Geometry check sheet. Reference: the model listing, model coordinates, mm. A direction names the side the tool comes from. Round coordinates to 2 decimals unless told otherwise and drop trailing zeros. Order: outer loops, then holes, each group sorted by start corner. A loop starts at its lowest first (then second) coordinate and runs counter-clockwise, first axis right, second up. Notation, with made-up numbers: (61, 88) - (108, 88) arc R10 cw to (108, 93) - close; hole circle Ø6 at (25.5, 6). An arc over 180 degrees is marked (long way). Answer as CSV lines item,"result". Start each with the question number.
```python
from build123d import *

# Parameters (mm, degrees)
F0_R     = 3.175
F1_DEPTH = 3.175
F2_R     = 1.5875
F3_DEPTH = 31.75
F4_R     = 3.175
F4_R_2   = 1.5875
F5_DEPTH = 3.175


with BuildPart() as f1:
    # F0 (on Front) → F1 (new body)
    with BuildSketch(Plane.XZ):
        Circle(F0_R)
    extrude(amount=F1_DEPTH)

    # F2 (on face) → F3 (join)
    with BuildSketch(Plane.XZ.offset(3.175)):
        Circle(F2_R)
    extrude(amount=F3_DEPTH)

    # F4 (on face) → F5 (join)
    with BuildSketch(Plane.XZ.offset(34.925)):
        Circle(F4_R)
        Circle(F4_R_2, mode=Mode.SUBTRACT)
        Circle(F4_R_2)
    extrude(amount=F5_DEPTH)


solid = f1.part
```
1. Thickness scan on probe 1 along Y at (x, z) = (-0.5, 1.75) (3 decimals); probe 2 along Z at (x, y) = (0, -11); probe 3 along Z at (x, y) = (1.25, -34). Record the ranges inside material, lowest first.
2. Section check A-A on x = 2.25. Record the boundary of the cut face in (y, z) (3 decimals).
3. Access from +Z, -Z, +X, -X, +Y, -Y to the whole of each face (thin tool, end or side, straight path). Record for faces 1 (the face through (-0.69, -36.49, -3.1)), 2 (the face through (1.4, -34.925, -1.4)).
4. Section check C-C on x = 0. Record the boundary of the cut face in (y, z) (1 decimal), plus the area to 3 significant figures.
5. Section check D-D on z = 0. Record the boundary of the cut face in (x, y) (1 decimal), plus the area to 3 significant figures.
6. Go/stop test with flat-tipped pins: pin 1 Ø3 at (y, z) = (-19, -1.5) entering from -X; pin 2 Ø2 at (x, y) = (1.5, -30.5) entering from +Z; pin 3 Ø1 at (y, z) = (-33, -1.5) entering from +X. Record where each tip stops, or that it passes through.
7. Draft check along Y on faces 3 (the face through (0, -38.1, 0)), 4 (the face through (1.4, -3.175, -1.4)), 5 (the face through (0, 0, 0)), 6 (the face through (-0.34, -18.83, -1.55)). Enter one of: released by +Y, released by -Y, zero draft, split by the parting line, or undercut.
8. Section check B-B on z = 2. Record the boundary of the cut face in (x, y) (3 decimals).
Numbers:
1,probe 1,"y = -38.1 to -34.925, -3.175 to 0"
1,probe 2,"z = -1.59 to 1.59"
1,probe 3,"z = -0.98 to 0.98"
2,outline,"(-38.1, -2.24) - (-34.925, -2.24) - (-34.925, 2.24) - (-38.1, 2.24) - close; (-3.175, -2.24) - (0, -2.24) - (0, 2.24) - (-3.175, 2.24) - close"
3,face 1,"+Y, -Y"
3,face 2,"none"
4,outline,"(-38.1, -3.2) - (-34.9, -3.2) - (-34.9, -1.6) - (-3.2, -1.6) - (-3.2, -3.2) - (0, -3.2) - (0, 3.2) - (-3.2, 3.2) - (-3.2, 1.6) - (-34.9, 1.6) - (-34.9, 3.2) - (-38.1, 3.2) - close"
4,area,"141 mm2"
5,outline,"(-3.2, -38.1) - (3.2, -38.1) - (3.2, -34.9) - (1.6, -34.9) - (1.6, -3.2) - (3.2, -3.2) - (3.2, 0) - (-3.2, 0) - (-3.2, -3.2) - (-1.6, -3.2) - (-1.6, -34.9) - (-3.2, -34.9) - close"
5,area,"141 mm2"
6,pin 1,"stops at x = -1.59"
6,pin 2,"stops at z = 1.51"
6,pin 3,"stops at x = 1.23"
7,face 3,"released by -Y"
7,face 4,"undercut"
7,face 5,"released by +Y"
7,face 6,"undercut"
8,outline,"(-2.466, -38.1) - (2.466, -38.1) - (2.466, -34.925) - (-2.466, -34.925) - close; (-2.466, -3.175) - (2.466, -3.175) - (2.466, 0) - (-2.466, 0) - close"
